The model under review builds one solid part; all positions refer to its coordinate system, in mm. A direction names the side the tool comes from. Coordinates: 2 decimals unless noted, no trailing zeros. Write each loop counter-clockwise with the first axis right and the second up, starting at its lowest first coordinate (ties: lowest second). Pieces come first, ordered by that corner, then holes.
1) Add section C-C, the plane z = 0. State the section outline as (x, y) points.
2) For P1, Ø3, axis at x = -20.86, y = 7, coming from the -Z side; P2, Ø1.5, axis at y = 9.5, z = 1, coming from the +X side, all flat-tipped, find the tip position at first contact; note any pin that passes through.
3) Mouldability with a two-part tool opening along X and no side actions: class faces 1 (the cylindrical face through (-18.497, -8.118, 0.021)), 2 (the cylindrical face through (-18.32, 10.28, -0.02)), 3 (the flat face through (-25, 0, 1.5)) as released by +X, released by -X, zero draft, split by the parting line, or undercut.
4) Add section D-D, the plane y = 7. State the section outline as (x, z) points, then the cut area to 3 significant figures.
5) Machinability: for faces 4 (the cylindrical face through (-18.497, 8.118, 0.021)), 5 (the flat face through (-25, 0, -1.5)), 6 (the cylindrical face through (-23.15, -6.45, 0.02)), which of the approach directions +Z, -Z, +X, -X, +Y, -Y give a long, thin tool a straight path to every point of the face, cutting with its end or side? Answer none if there is none.
6) For line 1 (Y direction, x = -19.75, z = 0); line 2 (Y direction, x = -19.5, z = 1.3); line 3 (Y direction, x = -22, z = 1.25), list the stretches that pass through material, from the lowest coordinate up.
7) Add section B-B, the plane x = -19.5. State the section outline as (y, z) points, then the cut area to 3 significant figures.
8) Add section A-A, the plane x = -18. State the section outline as (y, z) points, then the cut area to 3 significant figures.
from build123d import *

# Parameters (mm, degrees)
SKETCH_1_R        = 1
EXTRUDE_1_DEPTH   = 1.5
EXTRUDE_1_2_DEPTH = 1.5
EXTRUDE_2_DEPTH   = 3
FILLET_1_R        = 1


with BuildPart() as part:
    # Sketch 1 → Extrude 1 (new body, symmetric)
    with BuildSketch(Plane.XY):
        with BuildLine():
            ThreePointArc((-20.819004975, 11.532954168), (-21.781247924, 9.592561643), (-22.563107092, 7.572727273))
            ThreePointArc((-22.563107092, 7.572727273), (-21.429380887, 5.293546522), (-19.150200137, 6.427272727))
            ThreePointArc((-19.150200137, 6.427272727), (-18.486605381, 8.141585932), (-17.669911786, 9.788473706))
            ThreePointArc((-17.669911786, 9.788473706), (-18.372218149, 12.235260532), (-20.819004975, 11.532954168))
        make_face()
        with Locations((-19.24445838, 10.660713937)):
            Circle(SKETCH_1_R, mode=Mode.SUBTRACT)
        with Locations((-20.856653615, 7)):
            Circle(SKETCH_1_R, mode=Mode.SUBTRACT)
    extrude(amount=EXTRUDE_1_DEPTH, both=True)



with BuildPart() as body_2:
    # Sketch 1 → Extrude 1 2 (new body, symmetric)
    with BuildSketch(Plane.XY):
        with BuildLine():
            ThreePointArc((-20.819004975, -11.532954168), (-21.781247924, -9.592561643), (-22.563107092, -7.572727273))
            ThreePointArc((-22.563107092, -7.572727273), (-21.429380887, -5.293546522), (-19.150200137, -6.427272727))
            ThreePointArc((-19.150200137, -6.427272727), (-18.486605381, -8.141585932), (-17.669911786, -9.788473706))
            ThreePointArc((-17.669911786, -9.788473706), (-18.372218149, -12.235260532), (-20.819004975, -11.532954168))
        make_face()
        with Locations((-19.24445838, -10.660713937)):
            Circle(SKETCH_1_R, mode=Mode.SUBTRACT)
        with Locations((-20.856653615, -7)):
            Circle(SKETCH_1_R, mode=Mode.SUBTRACT)
    extrude(amount=EXTRUDE_1_2_DEPTH, both=True)


with BuildPart() as part_1:
    add(part.part)

    add(body_2.part)  # Extrude 2 merges body 2
    # Sketch 2 → Extrude 2 (add)
    with BuildSketch(Plane.XY.offset(1.5)):
        with BuildLine():
            Line((-19.24445838, 12.460713937), (-23.387616556, 12.460713937))
            ThreePointArc((-23.387616556, 12.460713937), (-26.5, 0), (-23.387616556, -12.460713937))
            Line((-23.387616556, -12.460713937), (-19.24445838, -12.460713937))
            ThreePointArc((-19.24445838, -12.460713937), (-20.158232856, -12.211525404), (-20.819004975, -11.532954168))
            ThreePointArc((-20.819004975, -11.532954168), (-21.781247924, -9.592561643), (-22.563107092, -7.572727273))
            ThreePointArc((-22.563107092, -7.572727273), (-22.646911391, -6.812978362), (-22.407893773, -6.086953468))
            ThreePointArc((-22.407893773, -6.086953468), (-23.162368256, -6.448682563), (-23.782272592, -5.886723226))
            ThreePointArc((-23.782272592, -5.886723226), (-24.5, 0), (-23.782272592, 5.886723226))
            ThreePointArc((-23.782272592, 5.886723226), (-23.162368256, 6.448682563), (-22.407893773, 6.086953468))
            ThreePointArc((-22.407893773, 6.086953468), (-22.646911391, 6.812978362), (-22.563107092, 7.572727273))
            ThreePointArc((-22.563107092, 7.572727273), (-21.781247924, 9.592561643), (-20.819004975, 11.532954168))
            ThreePointArc((-20.819004975, 11.532954168), (-20.158232856, 12.211525404), (-19.24445838, 12.460713937))
        make_face()
    extrude(amount=-EXTRUDE_2_DEPTH)

    # Fillet 1
    fillet_1_edges = [part_1.edges().sort_by_distance(p)[0] for p in [
        (-23.387616556, -12.460713937, 0),
        (-23.387616556, 12.460713937, 0),
    ]]
    fillet(fillet_1_edges, radius=FILLET_1_R)


solid = part_1.part
Geometry results:
1. outline: (-23.78, -5.89) arc R24.5 cw to (-23.78, 5.89) arc R0.75 cw to (-22.41, 6.09) arc R1.8 ccw to (-19.15, 6.43) arc R20.2 cw to (-17.67, 9.79) arc R1.8 ccw to (-19.24, 12.46) - (-22.78, 12.46) arc R1 ccw to (-23.67, 11.91) arc R26.5 ccw to (-23.67, -11.91) arc R1 ccw to (-22.78, -12.46) - (-19.24, -12.46) arc R1.8 ccw to (-17.67, -9.79) arc R20.2 cw to (-19.15, -6.43) arc R1.8 ccw to (-22.41, -6.09) arc R0.75 cw to start; hole circle Ø2 at (-20.86, -7); hole circle Ø2 at (-20.86, 7); hole circle Ø2 at (-19.24, -10.66); hole circle Ø2 at (-19.24, 10.66)
2. P1: stops at z = -1.5
2. P2: stops at x = -17.49
3. face 1: released by +X
3. face 2: undercut
3. face 3: zero draft
4. outline: (-25.56, -1.5) - (-21.86, -1.5) - (-21.86, 1.5) - (-25.56, 1.5) - close; (-19.86, -1.5) - (-18.95, -1.5) - (-18.95, 1.5) - (-19.86, 1.5) - close
4. area: 13.8 mm2
5. face 4: +Z, -Z, +X
5. face 5: -Z, +X, -X, +Y, -Y
5. face 6: +Z, -Z
6. line 1: y = -12.46 to -11.52, -9.8 to -5.58, 5.58 to 9.8, 11.52 to 12.46
6. line 2: y = -12.46 to -11.63, -9.69 to -5.82, 5.82 to 9.69, 11.63 to 12.46
6. line 3: y = -12.46 to -5.61, 5.61 to 12.46
7. outline: (-12.46, -1.5) - (-11.63, -1.5) - (-11.63, 1.5) - (-12.46, 1.5) - close; (-9.69, -1.5) - (-5.82, -1.5) - (-5.82, 1.5) - (-9.69, 1.5) - close; (5.82, -1.5) - (9.69, -1.5) - (9.69, 1.5) - (5.82, 1.5) - close; (11.63, -1.5) - (12.46, -1.5) - (12.46, 1.5) - (11.63, 1.5) - close
7. area: 28.3 mm2
8. outline: (-11.96, -1.5) - (-9.17, -1.5) - (-9.17, 1.5) - (-11.96, 1.5) - close; (9.17, -1.5) - (11.96, -1.5) - (11.96, 1.5) - (9.17, 1.5) - close
8. area: 16.8 mm2
